The listing builds one solid part. Answer for the finished solid, in the listing's coordinates (mm). Face numbers are marked on the shaded views. A direction names the side the tool comes from. Round coordinates to 2 decimals unless told otherwise and drop trailing zeros. Write each loop counter-clockwise with the first axis right and the second up, starting at its lowest first coordinate (ties: lowest second). Pieces come first, ordered by that corner, then holes. Notation, with made-up numbers: M -37,82.25 L -4,82.25 A22 ccw -4,108.25 Z; hole C 38,24 d6. An arc over 180 degrees is marked long. Write each question's results on one line, items separated by ' | '.
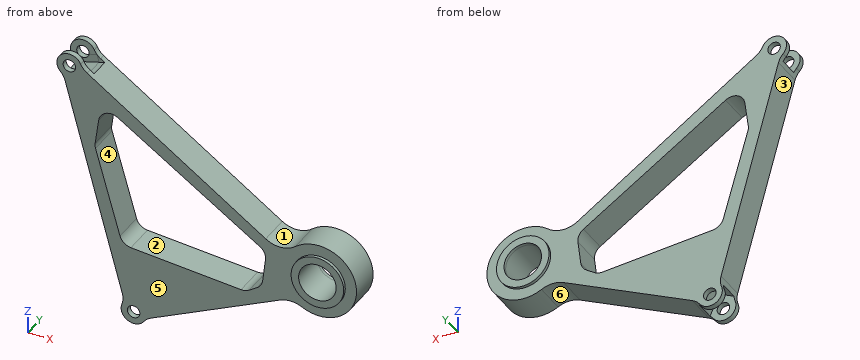
from build123d import *

# Parameters (mm, degrees)
F0_R           = 10
F0_R_2         = 30
F1_DEPTH       = 50
F3_W           = 32
F3_H           = 46.9773098714
F4_DEPTH       = 36
F4_DEPTH_BACK  = 36
F7_W           = 64.344675952
F7_H           = 32
F8_DEPTH       = 35
F8_DEPTH_BACK  = 25
F10_DEPTH      = 100
F11_R          = 20
F12_R          = 42
F12_R_2        = 30
F13_DEPTH      = 5
F14_R          = 42
F14_R_2        = 30
F15_DEPTH      = 5
F16_W          = 32
F16_H          = 12.6297663026
F17_DEPTH      = 25
F17_DEPTH_BACK = 25


# Not quite as in the source:
# - a feature names something its author has since deleted; it is built from what else it names


with BuildPart() as f1:
    # F0 (on Front) → F1 (new body)
    with BuildSketch(Plane.XZ):
        with BuildLine():
            ThreePointArc((-62.5780437897, -52.7205259787), (-44.9107725801, -48.9739327439), (-27.3963571385, -53.3801425208))
            ThreePointArc((-27.3963571385, -53.3801425208), (59.6815194776, 6.173834533), (-37.7432491465, 46.6416889045))
            ThreePointArc((-37.7432491465, 46.6416889045), (-61.1526251037, 37.7745700431), (-85.2484645361, 44.5580206149))
            Line((-85.2484645361, 44.5580206149), (-370.7956962097, 236.8532567171))
            ThreePointArc((-370.7956962097, 236.8532567171), (-376.7925336048, 242.1856420807), (-381.1612781983, 248.9169467897))
            ThreePointArc((-381.1612781983, 248.9169467897), (-410.6071858154, 256.8281563435), (-413.6417851947, 226.4894035906))
            ThreePointArc((-413.6417851947, 226.4894035906), (-409.1637807856, 220.5019975774), (-406.3054242786, 213.5932095263))
            Line((-406.3054242786, 213.5932095263), (-314.4991596079, -121.5832610972))
            ThreePointArc((-314.4991596079, -121.5832610972), (-313.4615655347, -130.8078667851), (-315.293607643, -139.9080631166))
            ThreePointArc((-315.293607643, -139.9080631166), (-305.9378740774, -164.4922463623), (-280.3150583777, -158.5438741459))
            ThreePointArc((-280.3150583777, -158.5438741459), (-275.1112486364, -152.9838392789), (-268.6751253171, -148.913220141))
            Line((-268.6751253171, -148.913220141), (-62.5780437897, -52.7205259787))
        make_face()
        with Locations((-296.5337380309, -146.8411210378)):
            Circle(F0_R, mode=Mode.SUBTRACT)
        Circle(F0_R_2, mode=Mode.SUBTRACT)
        with Locations((-399.2431908367, 240.3703430585)):
            Circle(F0_R, mode=Mode.SUBTRACT)
    extrude(amount=F1_DEPTH)

    # F3 (on face) → F4 (cut, two sides)
    with BuildSketch(Plane(origin=(-323.5290376394, 0, -88.6159831057), x_dir=(0, -1, 0), z_dir=(-0.9644750818, 0, -0.2641738379))) as f4_sk:
        with Locations((25, 344.0173126814)):
            Rectangle(F3_W, F3_H)
    extrude(amount=F4_DEPTH, mode=Mode.SUBTRACT)
    extrude(f4_sk.sketch, amount=-F4_DEPTH_BACK, mode=Mode.SUBTRACT)

    # F7 (on offset) → F8 (cut, two sides)
    with BuildSketch(Plane(origin=(9.0113675019, 0, -19.3072515422), x_dir=(0.9061594556, 0, 0.422936214), z_dir=(0.422936214, 0, -0.9061594556))) as f8_sk:
        with Locations((-346.1694030438, 25)):
            Rectangle(F7_W, F7_H)
    extrude(amount=-F8_DEPTH, mode=Mode.SUBTRACT)
    extrude(f8_sk.sketch, amount=F8_DEPTH_BACK, mode=Mode.SUBTRACT)

    # F9 (on face) → F10 (cut)
    with BuildSketch(Plane.XZ.offset(50)):
        Polygon((-348.2052087784, 193.6148256063), (-358.6101531982, 116.7783439159), (-314.4991596079, -37.6950278878), (-117.6957413554, -55.3033873439), (-91.2832021713, -37.6950278878), (-84.079772234, 21.5331036597), align=None)
    extrude(amount=-F10_DEPTH, mode=Mode.SUBTRACT)

    # F11
    f11_edges = [f1.edges().sort_by_distance(p)[0] for p in [
        (-348.205209, -25, 193.614826),
        (-358.610153, -25, 116.778344),
        (-84.079772, -25, 21.533104),
        (-91.283202, -25, -37.695028),
        (-117.695741, -25, -55.303387),
        (-314.49916, -25, -37.695028),
    ]]
    fillet(f11_edges, radius=F11_R)

    # F12 (on face) → F13 (join)
    with BuildSketch(Plane.XZ.offset(50)):
        Circle(F12_R)
        Circle(F12_R_2, mode=Mode.SUBTRACT)
    extrude(amount=F13_DEPTH)

    # F14 (on face) → F15 (join)
    with BuildSketch(Plane(origin=(0, 0, 0), x_dir=(-1, 0, 0), z_dir=(0, 1, 0))):
        Circle(F14_R)
        Circle(F14_R_2, mode=Mode.SUBTRACT)
    extrude(amount=F15_DEPTH)

    # F16 (on face) → F17 (cut, two sides)
    with BuildSketch(Plane(origin=(-288.8079346956, 0, -79.1057249405), x_dir=(0, -1, 0), z_dir=(-0.9644750818, 0, -0.2641738379))) as f17_sk:
        with Locations((25, 326.843540897)):
            Rectangle(F16_W, F16_H)
    extrude(amount=F17_DEPTH, mode=Mode.SUBTRACT)
    extrude(f17_sk.sketch, amount=-F17_DEPTH_BACK, mode=Mode.SUBTRACT)


solid = f1.part
1) Find the intervals of material crossed by line 1 (X direction, y = -36, z = -26.5); line 2 (X direction, y = -36, z = 23); line 3 (Y direction, x = -66.5, z = -6), in increasing order.
Return value:
line 1: -340.54 to -317.58, -89.92 to -14.06, 14.06 to 53.83 | line 2: -354.1 to -331.83, -89.02 to -19.26, 19.26 to 55.42 | line 3: -50 to 0
2) Section C-C (z = 0) is taken. Determine the outline of the cut face in (x, y), then the cut area to 3 significant figures.
Return value:
outline: M -347.8,-50 L -325.26,-50 L -325.26,0 L -347.8,0 Z; M -86.7,-50 L -42,-50 L -42,-55 L -30,-55 L -30,5 L -42,5 L -42,0 L -86.7,0 Z; M 30,-55 L 42,-55 L 42,-50 L 60,-50 L 60,0 L 42,0 L 42,5 L 30,5 Z | area: 5,700 mm²
3) Each of these flat-tipped pins is pushed along its axis until it touches: pin 1 (6 mm diameter, centred on x = -373, z = 233.5, fed in from -Y); pin 2 (10 mm diameter, centred on x = -45, y = -36, fed in from -Z); pin 3 (8 mm diameter, centred on y = -20, z = 80, fed in from +X); pin 4 (18 mm diameter, centred on x = -399.24, z = 240.37, fed in from -Y). Where does it stop, or does it pass through?
Return value:
pin 1: y = -50 | pin 2: z = -49.37 | pin 3: x = -131.94 | pin 4: through
4) Section B-B (y = -31) is taken. Determine the outline of the cut face in (x, z), then the cut area to 3 significant figures.
Return value:
outline: M -409.05,220.3 A30 cw -406.31,213.59 L -314.5,-121.58 A30 cw -313.48,-131.2 L -290.32,-120.39 L -275.11,-152.98 A30 cw -268.68,-148.91 L -62.58,-52.72 A40 cw -27.4,-53.38 A60 ccw long -37.74,46.64 A40 cw -85.25,44.56 L -364.38,232.53 Z; hole M -358.05,120.93 A20 ccw -357.46,112.75 L -318.27,-24.49 A20 ccw -300.82,-38.92 L -124.71,-54.68 A20 ccw -111.84,-51.4 L -98.93,-42.79 A20 ccw -90.17,-28.57 L -85.58,9.16 A20 ccw -94.52,28.34 L -321.71,176.35 A20 ccw -352.45,162.28 Z; hole C 0,0 d60 | area: 42,600 mm²
5) The mould has two halves that part along X. Classify the marked faces 3, 4, 5 and 6: +X half, -X half, draft (parallel to the pull), parting line (faces both ways), or undercut.
Return value:
face 3: -X half | face 4: undercut | face 5: draft | face 6: undercut
6) Section A-A (x = 0) is taken. Determine the outline of the cut face in (y, z), then the cut area to 3 significant figures.
Return value:
outline: M -55,-42 L -50,-42 L -50,-60 L 0,-60 L 0,-42 L 5,-42 L 5,-30 L -55,-30 Z; M -55,30 L 5,30 L 5,42 L 0,42 L 0,60 L -50,60 L -50,42 L -55,42 Z | area: 3,240 mm²
7) A tool of negligible diameter and unlimited length cuts with its end or side. For the marked faces 1 and 2, from which of +Z, -Z, +X, -X, +Y, -Y can it reach the whole face along a straight path? Write none if from no direction.
Return value:
face 1: +Z, +Y, -Y | face 2: +Y, -Y
8) Section D-D (z = -69.5) is taken. Determine the outline of the cut face in (x, y).
Return value:
outline: M -328.76,-50 L -98.53,-50 L -98.53,0 L -328.76,0 Z
